from build123d import *


with BuildPart() as part:
    # Sketch1 → Revolve1 (revolve)
    with BuildSketch(Plane(origin=(0, 0, 0), x_dir=(0, 0, -1), z_dir=(1, 0, 0))):
        with BuildLine():
            Line((0, 0), (0, 14.75))
            Line((0, 14.75), (27.299792462, 14.75))
            ThreePointArc((27.299792462, 14.75), (27.873368898, 14.930847956), (28.239485083, 15.407979857))
            Line((28.239485083, 15.407979857), (32.67411308, 27.592020143))
            ThreePointArc((32.67411308, 27.592020143), (33.040229264, 28.069152044), (33.613805701, 28.25))
            Line((33.613805701, 28.25), (42.513598163, 28.25))
            Line((42.513598163, 28.25), (42.513598163, 24.25))
            ThreePointArc((42.513598163, 24.25), (49.544009667, 13.019738091), (52, 0))
            Line((52, 0), (0, 0))
        make_face()
    revolve(axis=Axis((0, 0, 0), (0, 0, -1)))


solid = part.part
Could you check a few things on this model? Use its own coordinates, in mm. A direction names the side the tool comes from. Give positions to 0.01 mm unless a question says otherwise; leave off trailing zeros. Write each loop counter-clockwise with the first axis right and the second up, starting at its lowest first coordinate (ties: lowest second). Pieces come first, ordered by that corner, then holes. Notation, with made-up numbers: (76.5, 88) -> (91.5, 88) arc R23 cw to (91.5, 125) -> close; hole circle Ø3 at (2.5, 45.25). An arc over 180 degrees is marked (long way). Answer as a JSON object with one key per item and string values.
Q1. Suppose I cut it at A-A on x = 0. Write out the boundary of the cut face in (y, z), then the cut area to 3 significant figures.
Taken from the geometry:
{"outline": "(-28.25, -42.51) -> (-24.25, -42.51) arc R35.74 ccw to (24.25, -42.51) -> (28.25, -42.51) -> (28.25, -33.61) arc R1 ccw to (27.59, -32.67) -> (15.41, -28.24) arc R1 cw to (14.75, -27.3) -> (14.75, 0) -> (-14.75, 0) -> (-14.75, -27.3) arc R1 cw to (-15.41, -28.24) -> (-27.59, -32.67) arc R1 ccw to (-28.25, -33.61) -> close", "area": "1,900 mm²"}
Q2. Which directions (+Z, -Z, +X, -X, +Y, -Y) give clear straight access to the entire face, cutting with the end or side of a thin tool? Please do faces 1 (the flat face through (21.1, 12.4, -42.514)), 2 (the cylindrical face through (23.82, 15.19, -38.13)), 3 (the cylindrical face through (4.43, 14.07, -13.84)).
Taken from the geometry:
{"face 1": "-Z", "face 2": "+Z, -Z", "face 3": "+Z"}
Q3. Will these pins go through, and if not, where does the flat tip stop? pin 1 Ø10 at (x, y) = (-19.5, 14) entering from -Z; pin 2 Ø12 at (y, z) = (-0.5, -31) entering from +X; pin 3 Ø8 at (y, z) = (-10, -34) entering from +X.
Taken from the geometry:
{"pin 1": "stops at z = -46.53", "pin 2": "stops at x = 28.25", "pin 3": "stops at x = 27.61"}
Q4. Suppose I cut it at C-C on z = -25. Write out the boundary of the cut face in (x, y), then the cut area to 3 significant figures.
Taken from the geometry:
{"outline": "circle Ø29.5 at (0, 0)", "area": "683 mm²"}
Q5. Please list where these lines run through material, in increasing order: L1, parallel to Z at x = 23.5, y = 2.5; L2, parallel to Z at x = -10.5, y = 6.5; L3, parallel to Y at x = 7, z = -40.
Taken from the geometry:
{"L1": "z = -43.07 to -31.23", "L2": "z = -49.8 to 0", "L3": "y = -27.37 to 27.37"}
